Read the model definition and answer for the solid it produces. Units are mm, in the model's axes. A direction names the side the tool comes from. Coordinates: 2 decimals unless noted, no trailing zeros. Loops run counter-clockwise (first coordinate to the right, second up) from the corner with the lowest first, then second, coordinate; pieces in that order, holes last. Notation, with made-up numbers: (8.25, 46) -> (27.25, 46) arc R21 cw to (27.25, 53) -> close; hole circle Ø3 at (-20.75, 63). An arc over 180 degrees is marked (long way). Answer in a Markdown table with one row per item.
```python
from build123d import *

# Parameters (mm, degrees)
SKETCH1_W           = 45
SKETCH1_H           = 55
BOSS_EXTRUDE1_DEPTH = 40
SKETCH2_R           = 5
CUT_EXTRUDE1_DEPTH  = 45
SKETCH3_W           = 70
SKETCH3_H           = 10
BOSS_EXTRUDE2_DEPTH = 20
SKETCH6_R           = 1.5
CUT_EXTRUDE3_DEPTH  = 10
BOSS_EXTRUDE4_DEPTH = 3
BOSS_EXTRUDE5_START = 10
BOSS_EXTRUDE5_DEPTH = 10


with BuildPart() as part:
    # Sketch1 → Boss-Extrude1 (new body)
    with BuildSketch(Plane(origin=(0, 0, 0), x_dir=(1, 0, 0), z_dir=(0, 1, 0))):
        Rectangle(SKETCH1_W, SKETCH1_H)
    extrude(amount=BOSS_EXTRUDE1_DEPTH)

    # Sketch2 → Cut-Extrude1 (cut)
    with BuildSketch(Plane(origin=(22.5, 0, 0), x_dir=(0, 0, -1), z_dir=(1, 0, 0))):
        with Locations((-17.5, 20)):
            Circle(SKETCH2_R)
    extrude(amount=-CUT_EXTRUDE1_DEPTH, mode=Mode.SUBTRACT)

    # Sketch3 → Boss-Extrude2 (add)
    with BuildSketch(Plane(origin=(0, 0, -27.5), x_dir=(-1, 0, 0), z_dir=(0, 0, -1))):
        with Locations((0, 20)):
            Rectangle(SKETCH3_W, SKETCH3_H)
    extrude(amount=BOSS_EXTRUDE2_DEPTH)

    # Sketch6 → Cut-Extrude3 (cut)
    with BuildSketch(Plane(origin=(0, 25, 0), x_dir=(1, 0, 0), z_dir=(0, 1, 0))):
        with Locations(Location((28.771358024, 37.5, 0), (0, 0, 180))):
            Circle(SKETCH6_R)
        with Locations(Location((-27.782656664, 37.5, 0), (0, 0, 180))):
            Circle(SKETCH6_R)
    extrude(amount=-CUT_EXTRUDE3_DEPTH, mode=Mode.SUBTRACT)

    # Sketch7 → Boss-Extrude4 (add)
    with BuildSketch(Plane(origin=(0, 25, 0), x_dir=(1, 0, 0), z_dir=(0, 1, 0))):
        with BuildLine():
            Line((18.533858024, 112.5), (14.933858024, 112.5))
            Line((14.933858024, 112.5), (13.262014547, 99.438722839))
            ThreePointArc((13.262014547, 99.438722839), (13.566755729, 98.09818866), (14.664816743, 97.271048355))
            ThreePointArc((14.664816743, 97.271048355), (21.67882772, 86.432675937), (12.161050226, 77.710372444))
            ThreePointArc((12.161050226, 77.710372444), (10.890055897, 77.186471223), (10.257494727, 75.965911745))
            Line((10.257494727, 75.965911745), (9.15513462, 67.353723404))
            Line((9.15513462, 67.353723404), (14.008858024, 62.5))
            ThreePointArc((14.008858024, 62.5), (21.079925836, 59.571067812), (24.008858024, 52.5))
            Line((24.008858024, 52.5), (24.008858024, 37.5))
            ThreePointArc((24.008858024, 37.5), (25.403761978, 34.132403955), (28.771358024, 32.7375))
            ThreePointArc((28.771358024, 32.7375), (32.138954069, 34.132403955), (33.533858024, 37.5))
            Line((33.533858024, 37.5), (33.533858024, 72.5))
            Line((33.533858024, 72.5), (18.533858024, 112.5))
        make_face()
    boss_extrude4 = extrude(amount=BOSS_EXTRUDE4_DEPTH)

    # Sketch8 → Boss-Extrude5 (add)
    with BuildSketch(Plane.XZ.offset(-25).offset(BOSS_EXTRUDE5_START)):
        with BuildLine():
            Line((33.533858024, -72.5), (14.008858024, -62.5))
            Line((14.008858024, -62.5), (9.15513462, -67.353723404))
            Line((9.15513462, -67.353723404), (10.257494727, -75.965911745))
            ThreePointArc((10.257494727, -75.965911745), (10.890055897, -77.186471223), (12.161050226, -77.710372444))
            ThreePointArc((12.161050226, -77.710372444), (21.67882772, -86.432675937), (14.664816743, -97.271048355))
            ThreePointArc((14.664816743, -97.271048355), (13.566755729, -98.09818866), (13.262014547, -99.438722839))
            Line((13.262014547, -99.438722839), (14.933858024, -112.5))
            Line((14.933858024, -112.5), (18.533858024, -112.5))
            Line((18.533858024, -112.5), (33.533858024, -72.5))
        make_face()
    extrude(amount=-BOSS_EXTRUDE5_DEPTH)

    # Mirror1: Boss-Extrude4 across plane
    add(boss_extrude4.mirror(Plane.ZX.offset(20)))


solid = part.part
```
1. A cutting plane is placed at C-C on x = -1.5. Give the vertices of the cut face in (y, z).
A:
| item | result |
|---|---|
| outline | (0, -27.5) -> (15, -27.5) -> (15, -47.5) -> (25, -47.5) -> (25, -27.5) -> (40, -27.5) -> (40, 27.5) -> (0, 27.5) -> close; hole circle Ø10 at (20, 17.5) |
2. A cutting plane is placed at B-B on z = 17.5. Give the vertices of the cut face in (x, y), and give its area (3 significant figures).
A:
| item | result |
|---|---|
| outline | (-22.5, 0) -> (22.5, 0) -> (22.5, 15) -> (-22.5, 15) -> close; (-22.5, 25) -> (22.5, 25) -> (22.5, 40) -> (-22.5, 40) -> close |
| area | 1,350 mm2 |
3. A tool of negligible diameter and unlimited length cuts with its end or side. For faces 4 (the flat face through (24.009, 26, -45)), 5 (the flat face through (33.534, 14, -55)), 6 (the flat face through (24, 28, -73)), 7 (the flat face through (28, 15, -60)), from which of +Z, -Z, +X, -X, +Y, -Y can it reach the whole face along a straight path? Write none if from no direction.
A:
| item | result |
|---|---|
| face 4 | +Z, -X, +Y |
| face 5 | +Z, -Z, +X, -Y |
| face 6 | -Z, +X, -X, +Y |
| face 7 | +X |
4. A cutting plane is placed at D-D on z = -34.5. Give the vertices of the cut face in (x, y), and give its area (3 significant figures).
A:
| item | result |
|---|---|
| outline | (-35, 15) -> (25.07, 15) -> (25.07, 12) -> (32.47, 12) -> (32.47, 15) -> (35, 15) -> (35, 25) -> (32.47, 25) -> (32.47, 28) -> (25.07, 28) -> (25.07, 25) -> (-35, 25) -> close |
| area | 744 mm2 |
5. Given pin 1 Ø2.5 at (y, z) = (13, -50) entering from +X; pin 2 Ø1 at (x, y) = (-23.5, 16) entering from +Z; pin 3 Ø6 at (x, z) = (11, -34) entering from +Y, each flat-ended and moving along its own axis, determine where each tip first touches the part or whether it passes through.
A:
| item | result |
|---|---|
| pin 1 | stops at x = 33.53 |
| pin 2 | stops at z = -27.5 |
| pin 3 | stops at y = 25 |
6. A cutting plane is placed at A-A on y = 20. Give the vertices of the cut face in (x, z).
A:
| item | result |
|---|---|
| outline | (-35, -47.5) -> (35, -47.5) -> (35, -27.5) -> (22.5, -27.5) -> (22.5, 12.5) -> (-22.5, 12.5) -> (-22.5, -27.5) -> (-35, -27.5) -> close; (-22.5, 22.5) -> (22.5, 22.5) -> (22.5, 27.5) -> (-22.5, 27.5) -> close; (9.16, -67.35) -> (10.26, -75.97) arc R2 ccw to (12.16, -77.71) arc R10 cw to (14.66, -97.27) arc R2 ccw to (13.26, -99.44) -> (14.93, -112.5) -> (18.53, -112.5) -> (33.53, -72.5) -> (14.01, -62.5) -> close; hole circle Ø3 at (-27.78, -37.5); hole circle Ø3 at (28.77, -37.5) |
7. The mould has two halves that part along Z. Classify faces 1 (the cylindrical face through (27.386, 20.07, -38.075)), 2 (the flat face through (35, 20, -37)), 3 (the flat face through (26.14, 20.11, -92.22)): pulls with the +Z half, pulls with the -Z half, needs draft (parallel to the pull), parting line crosses it, or undercut.
A:
| item | result |
|---|---|
| face 1 | undercut |
| face 2 | needs draft |
| face 3 | pulls with the -Z half |
8. Find the intervals of material crossed by probe 1 along Y at (x, z) = (-5, 17.5); probe 2 along Z at (x, y) = (-14.5, 9); probe 3 along X at (y, z) = (22, -22.5), in increasing order.
A:
| item | result |
|---|---|
| probe 1 | y = 0 to 15, 25 to 40 |
| probe 2 | z = -27.5 to 27.5 |
| probe 3 | x = -22.5 to 22.5 |
